Read the model definition and answer for the solid it produces. Units are mm, in the model's axes. A direction names the side the tool comes from. Round coordinates to 2 decimals unless told otherwise and drop trailing zeros. Loops run counter-clockwise (first coordinate to the right, second up) from the corner with the lowest first, then second, coordinate; pieces in that order, holes last. Notation, with made-up numbers: (10.5, -4.75) - (64.5, -4.75) arc R13 ccw to (64.5, 2.25) - close; hole circle Ø11 at (38.5, 22). An arc over 180 degrees is marked (long way). Use one line per item in the form item = value. Start each with the question number.
```python
from build123d import *

# Parameters (mm, degrees)
SKETCH1_W               = 95
SKETCH1_H               = 50
BOSS_EXTRUDE1_DEPTH     = 20
SKETCH4_R               = 1.425
CUT_EXTRUDE3_DEPTH      = 58.282196187
LPATTERN1_COUNT         = 2
LPATTERN1_PITCH         = 36
SKETCH5_R               = 1.5
CUT_EXTRUDE4_DEPTH      = 58.282196187
SKETCH6_W               = 5
SKETCH6_H               = 15
BOSS_EXTRUDE2_DEPTH     = 2
SKETCH7_W               = 76
SKETCH7_H               = 15
BOSS_EXTRUDE3_DEPTH     = 2
SHELL1_START            = 2
SHELL1_OUTLINE_W        = 91
SHELL1_OUTLINE_H        = 46
SHELL1_OUTLINE_R        = 3.5
SHELL1_OUTLINE_R_2      = 3.425
SHELL1_DEPTH            = 18
SHELL1_START_2          = 4.5
SHELL1_2_OUTLINE_W      = 1
SHELL1_2_OUTLINE_H      = 4
SHELL1_2_DEPTH          = 11
SKETCH2_R               = 3.35
CUT_EXTRUDE1_DEPTH      = 72.807033082
CUT_EXTRUDE5_DEPTH      = 75.647505009
CUT_EXTRUDE5_DEPTH_BACK = 75.647505009
SKETCH10_R              = 1.425


# Read off the part's stored shape, not the designer's step: Shell1
with BuildPart() as part:
    # Sketch1 → Boss-Extrude1 (new body)
    with BuildSketch(Plane.XY):
        Rectangle(SKETCH1_W, SKETCH1_H)
    extrude(amount=BOSS_EXTRUDE1_DEPTH)

    # Sketch4 → Cut-Extrude3 (cut, through all)
    with BuildSketch(Plane(origin=(0, 0, 0), x_dir=(-1, 0, 0), z_dir=(0, 0, -1))):
        with Locations((15.5, 8.25)):
            Circle(SKETCH4_R)
    cut_extrude3 = extrude(amount=-CUT_EXTRUDE3_DEPTH, mode=Mode.SUBTRACT)

    # LPattern1: Cut-Extrude3 ×2
    with Locations(*[(i * LPATTERN1_PITCH, 0, 0) for i in range(1, LPATTERN1_COUNT)]):
        add(cut_extrude3, mode=Mode.SUBTRACT)

    # Sketch5 → Cut-Extrude4 (cut, through all)
    with BuildSketch(Plane(origin=(0, 0, 0), x_dir=(-1, 0, 0), z_dir=(0, 0, -1))):
        with Locations((-32.5, -10)):
            Circle(SKETCH5_R)
        with Locations((32.5, -10)):
            Circle(SKETCH5_R)
    extrude(amount=-CUT_EXTRUDE4_DEPTH, mode=Mode.SUBTRACT)

    # Sketch6 → Boss-Extrude2 (add)
    with BuildSketch(Plane.XZ.offset(25)):
        with Locations((35.5, 10)):
            Rectangle(SKETCH6_W, SKETCH6_H)
    boss_extrude2 = extrude(amount=BOSS_EXTRUDE2_DEPTH)

    # Mirror1: Boss-Extrude2 across plane
    add(boss_extrude2.mirror(Plane(origin=(0, 0, 0), x_dir=(0, 0, 1), z_dir=(1, 0, 0))))

    # Sketch7 → Boss-Extrude3 (add)
    with BuildSketch(Plane.XZ.offset(27)):
        with Locations((0, 10)):
            Rectangle(SKETCH7_W, SKETCH7_H)
    extrude(amount=BOSS_EXTRUDE3_DEPTH)

    # Shell1 outline → Shell1 (cut)
    with BuildSketch(Plane.XY.offset(SHELL1_START)):
        Rectangle(SHELL1_OUTLINE_W, SHELL1_OUTLINE_H)
        with Locations((-32.5, -10)):
            Circle(SHELL1_OUTLINE_R, mode=Mode.SUBTRACT)
        with Locations((32.5, -10)):
            Circle(SHELL1_OUTLINE_R, mode=Mode.SUBTRACT)
        with Locations((-15.5, 8.25)):
            Circle(SHELL1_OUTLINE_R_2, mode=Mode.SUBTRACT)
        with Locations((20.5, 8.25)):
            Circle(SHELL1_OUTLINE_R_2, mode=Mode.SUBTRACT)
    extrude(amount=SHELL1_DEPTH, mode=Mode.SUBTRACT)

    # Shell1 2 outline → Shell1 2 (cut)
    with BuildSketch(Plane.XY.offset(SHELL1_START_2)):
        with Locations((-35.5, -25)):
            Rectangle(SHELL1_2_OUTLINE_W, SHELL1_2_OUTLINE_H)
        with Locations((35.5, -25)):
            Rectangle(SHELL1_2_OUTLINE_W, SHELL1_2_OUTLINE_H)
    extrude(amount=SHELL1_2_DEPTH, mode=Mode.SUBTRACT)

    # Sketch2 → Cut-Extrude1 (cut, through all)
    with BuildSketch(Plane.XZ.offset(25)):
        with Locations((-26.3, 10)):
            Circle(SKETCH2_R)
        with Locations((26.3, 10)):
            Circle(SKETCH2_R)
    extrude(amount=-CUT_EXTRUDE1_DEPTH, mode=Mode.SUBTRACT)

    # Sketch10 → Cut-Extrude5 (cut, two sides: drawn at the far end of the back side and taken through both)
    with BuildSketch(Plane.XZ.offset(29).offset(-CUT_EXTRUDE5_DEPTH_BACK)):
        with Locations((26.3, 10)):
            Circle(SKETCH10_R)
        with Locations((-26.3, 10)):
            Circle(SKETCH10_R)
    extrude(amount=CUT_EXTRUDE5_DEPTH + CUT_EXTRUDE5_DEPTH_BACK, mode=Mode.SUBTRACT)


solid = part.part
```
1) For faces 1 (the cylindrical face through (29.65, -10.03, 9.97)), 2 (the flat face through (-1, -28, 17.5)), 3 (the flat face through (35, -25, 10)), 4 (the cylindrical face through (17.08, 8.4, 10.87)), determine the directions among +Z, -Z, +X, -X, +Y, -Y from which every point of the face is accessible in a straight line to the end or side of a thin tool.
2) Straight lines are drawn through the part: line 1 (Y direction, x = -15.5, z = 8.25) (3 decimals); line 2 (Y direction, x = 32.5, z = 13); line 3 (X direction, y = 8, z = 3.75). For each, find the intervals that lie inside material, in ascending order. Write a range as from..to.
3) A cutting plane is placed at C-C on x = -3.5. Write down the section's boundary in (y, z), plus the area to 3 significant figures.
4) Flat-ended cylindrical pins translate along their axes: pin 1 (4 mm diameter, centred on x = -37.5, y = -18, fed in from +Z); pin 2 (6 mm diameter, centred on x = -26.3, z = 10, fed in from +Y); pin 3 (4.5 mm diameter, centred on y = -28, z = 9, fed in from -X). Find the tip coordinate at first contact, or state that the pin passes through.
5) A cutting plane is placed at D-D on x = -15.5. Write down the section's boundary in (y, z) (3 decimals).
6) A cutting plane is placed at B-B on y = -10. Write down the section's boundary in (x, z), plus the area to 3 significant figures.
7) Determine the mould class of faces 5 (the flat face through (-4, -24, 20)), 6 (the flat face through (-36, -25, 10)) for opening direction Y: +Y half, -Y half, draft (parallel to the pull), parting line (faces both ways), or undercut.
8) A cutting plane is placed at A-A on z = 16.5. Count the separate pieces of the cut face and the enclosed holes in it, plus the area to 3 significant figures.
Checks:
q1.face_1 = +Y
q1.face_2 = +Z, +X, -X, -Y
q1.face_3 = none
q1.face_4 = +Z
q2.line_1 = -29..-27, -25..-23, 4.825..6.825, 9.675..11.675, 23..25
q2.line_2 = -29..-27, -25..-23, -13.5..-11.5, -8.5..-6.5, 23..25
q2.line_3 = -47.5..-45.5, -18.92..-16.9, -14.1..-12.08, 17.08..19.1, 21.9..23.92, 45.5..47.5
q3.outline = (-29, 2.5) - (-27, 2.5) - (-27, 17.5) - (-29, 17.5) - close; (-25, 0) - (25, 0) - (25, 20) - (23, 20) - (23, 2) - (-23, 2) - (-23, 20) - (-25, 20) - close
q3.area = 202 mm²
q4.pin_1 = 2
q4.pin_2 = -27
q4.pin_3 = -38
q5.outline = (-29, 2.5) - (-27, 2.5) - (-27, 17.5) - (-29, 17.5) - close; (-25, 0) - (6.825, 0) - (6.825, 20) - (4.825, 20) - (4.825, 2) - (-23, 2) - (-23, 20) - (-25, 20) - close; (9.675, 0) - (25, 0) - (25, 20) - (23, 20) - (23, 2) - (11.675, 2) - (11.675, 20) - (9.675, 20) - close
q6.outline = (-47.5, 0) - (-34, 0) - (-34, 20) - (-36, 20) - (-36, 2) - (-45.5, 2) - (-45.5, 20) - (-47.5, 20) - close; (-31, 0) - (31, 0) - (31, 20) - (29, 20) - (29, 11.98) arc R3.35 cw to (29, 8.02) - (29, 2) - (-29, 2) - (-29, 8.02) arc R3.35 cw to (-29, 11.98) - (-29, 20) - (-31, 20) - close; (34, 0) - (47.5, 0) - (47.5, 20) - (45.5, 20) - (45.5, 2) - (36, 2) - (36, 20) - (34, 20) - close
q6.area = 390 mm²
q7.face_5 = draft
q7.face_6 = undercut
q8.separate_pieces = 5
q8.enclosed_holes = 6
q8.area = 860 mm²
